```python
from build123d import *

# Parameters (mm, degrees)
F0_R     = 10
F0_R_2   = 6
F1_DEPTH = 10
F2_R     = 2
F3_DEPTH = 64.001
F4_DEPTH = 3


with BuildPart() as f1:
    # F0 (on Front) → F1 (new body)
    with BuildSketch(Plane.XZ):
        Polygon((0, 64), (-100, 64), (-100, 54), (-80, 54), (-80, 0), (-20, 0), (-20, 54), (0, 54), align=None)
        with Locations((-50, 32)):
            Circle(F0_R, mode=Mode.SUBTRACT)
        with Locations((-50, 32)):
            Circle(F0_R)
        with Locations((-50, 32)):
            Circle(F0_R_2, mode=Mode.SUBTRACT)
    extrude(amount=F1_DEPTH)

    # F2 (on face) → F3 (cut, through all)
    with BuildSketch(Plane.XY.offset(64)):
        with Locations((-95, -5)):
            Circle(F2_R)
        with Locations((-5, -5)):
            Circle(F2_R)
    extrude(amount=-F3_DEPTH, mode=Mode.SUBTRACT)

    # F0 (on Front) → F4 (cut)
    with BuildSketch(Plane.XZ):
        with Locations((-50, 32)):
            Circle(F0_R)
        with Locations((-50, 32)):
            Circle(F0_R_2, mode=Mode.SUBTRACT)
    extrude(amount=F4_DEPTH, mode=Mode.SUBTRACT)


solid = f1.part
```
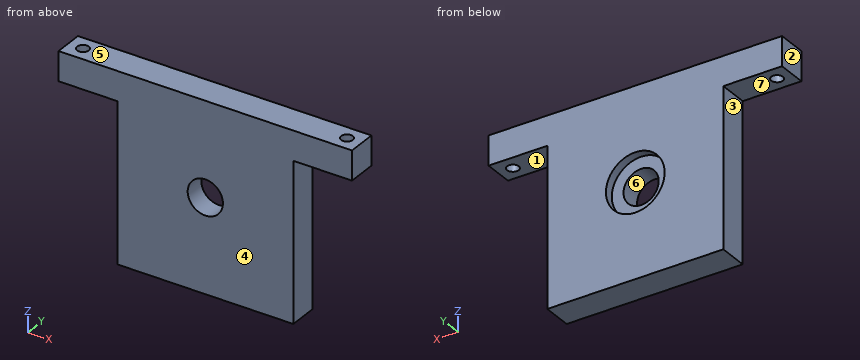
The listing builds one solid part. Answer for the finished solid, in the listing's coordinates (mm). Face numbers are marked on the shaded views. A direction names the side the tool comes from. Round coordinates to 2 decimals unless told otherwise and drop trailing zeros. Write each loop counter-clockwise with the first axis right and the second up, starting at its lowest first coordinate (ties: lowest second). Pieces come first, ordered by that corner, then holes. Notation, with made-up numbers: (86.25, -28) -> (110.25, -28) arc R21 ccw to (110.25, -4) -> close; hole circle Ø8 at (-4, 71). An arc over 180 degrees is marked (long way). Write item = value, one per line.
1) Section B-B on x = -51.5 is taken. Write down the section's boundary in (y, z), plus the area to 3 significant figures.
Check values:
outline = (-10, 0) -> (0, 0) -> (0, 22.11) -> (-3, 22.11) -> (-3, 26.19) -> (-10, 26.19) -> close; (-10, 37.81) -> (-3, 37.81) -> (-3, 41.89) -> (0, 41.89) -> (0, 64) -> (-10, 64) -> close
area = 499 mm²
2) Straight lines are drawn through the part: line 1 along Z through (x, y) = (-42, -2.5); line 2 along Y through (x, z) = (-95, 56.75); line 3 along Z through (x, y) = (-50, -1.3). For each, find the intervals that lie inside material, in ascending order. Write a range as [from, to].
Check values:
line_1 = [0, 26], [38, 64]
line_2 = [-10, -7], [-3, 0]
line_3 = [0, 22], [42, 64]
3) Section D-D on x = -95 is taken. Write down the section's boundary in (y, z).
Check values:
outline = (-10, 54) -> (-7, 54) -> (-7, 64) -> (-10, 64) -> close; (-3, 54) -> (0, 54) -> (0, 64) -> (-3, 64) -> close
4) For a pull along Z with two mould halves and no side action, classify the marked faces 4, 5, 6 and 7 as released by +Z, released by -Z, zero draft, split by the parting line, or undercut.
Check values:
face_4 = zero draft
face_5 = released by +Z
face_6 = undercut
face_7 = released by -Z
5) Which of the six approach directions +Z, -Z, +X, -X, +Y, -Y give full straight-line access (tool end or side, diameter ignored) to the marked faces 1, 2 and 3?
Check values:
face_1 = -Z, +X, +Y, -Y
face_2 = +Z, -Z, -X, +Y, -Y
face_3 = -Z, -X, +Y, -Y
6) Given pin 1 (3 mm diameter, centred on y = -7, z = 15.5, fed in from +X); pin 2 (4 mm diameter, centred on x = -15.5, y = -2, fed in from -Z); pin 3 (2.5 mm diameter, centred on x = -95, y = -5, fed in from -Z) (1 decimal); pin 4 (6 mm diameter, centred on x = -51.5, z = 28, fed in from +Y), each flat-ended and moving along its own axis, determine where each tip first touches the part or whether it passes through.
Check values:
pin_1 = -20
pin_2 = 54
pin_3 = through
pin_4 = -3
7) Section C-C on z = 32 is taken. Write down the section's boundary in (x, y).
Check values:
outline = (-80, -10) -> (-56, -10) -> (-56, -3) -> (-60, -3) -> (-60, 0) -> (-80, 0) -> close; (-44, -10) -> (-20, -10) -> (-20, 0) -> (-40, 0) -> (-40, -3) -> (-44, -3) -> close
8) Section A-A on y = -5 is taken. Write down the section's boundary in (x, z).
Check values:
outline = (-100, 54) -> (-97, 54) -> (-97, 64) -> (-100, 64) -> close; (-93, 54) -> (-80, 54) -> (-80, 0) -> (-20, 0) -> (-20, 54) -> (-7, 54) -> (-7, 64) -> (-93, 64) -> close; (-3, 54) -> (0, 54) -> (0, 64) -> (-3, 64) -> close; hole circle Ø12 at (-50, 32)
